Can you work these out from the model? Positions are in its coordinate system, mm. Round coordinates to 2 decimals unless told otherwise and drop trailing zeros. Loops run counter-clockwise (first coordinate to the right, second up) from the corner with the lowest first, then second, coordinate; pieces in that order, holes last. Notation, with made-up numbers: (83.5, -35) - (120.5, -35) arc R27 ccw to (120.5, -9) - close; hole circle Ø4 at (-3.75, 5). An arc over 180 degrees is marked (long way). Answer as CSV lines item,"result".
```python
from build123d import *

# Parameters (mm, degrees)
BOSS_EXTRUDE1_DEPTH   = 10.16
SKETCH2_W             = 76.2
SKETCH2_H             = 10.16
CUT_EXTRUDE1_DEPTH    = 4.572
CHAMFER1_SIZE         = 38.1
CHAMFER1_SIZE2        = 65.991135768
CHAMFER1_PART_2_SIZE  = 38.1
CHAMFER1_PART_2_SIZE2 = 65.991135768
FILLET1_R             = 25.4


with BuildPart() as part:
    # Sketch1 → Boss-Extrude1 (new body)
    with BuildSketch(Plane(origin=(0, 0, 0), x_dir=(0, 0, -1), z_dir=(1, 0, 0))):
        Polygon((-212.802604436, 0), (-212.802604436, 254), (-212.802604436, 279.4), (213.917395564, 279.4), (213.917395564, 254), (213.917395564, 0), (213.917395564, -50.8), (-212.802604436, -50.8), align=None)
        with BuildLine():
            Line((-95.25, 234.95), (95.25, 234.95))
            ThreePointArc((95.25, 234.95), (114.3, 215.9), (95.25, 196.85))
            Line((95.25, 196.85), (-95.25, 196.85))
            ThreePointArc((-95.25, 196.85), (-114.3, 215.9), (-95.25, 234.95))
        make_face(mode=Mode.SUBTRACT)
    extrude(amount=-BOSS_EXTRUDE1_DEPTH)

    # Sketch2 → Cut-Extrude1 (cut)
    with BuildSketch(Plane(origin=(0, 0, 0), x_dir=(0, 0, -1), z_dir=(1, 0, 0))):
        with Locations((-158.192604436, 127)):
            Rectangle(SKETCH2_W, SKETCH2_H)
        with Locations((0.557395564, 127)):
            Rectangle(SKETCH2_W, SKETCH2_H)
        with Locations((159.307395564, 127)):
            Rectangle(SKETCH2_W, SKETCH2_H)
    extrude(amount=-CUT_EXTRUDE1_DEPTH, mode=Mode.SUBTRACT)

    # Chamfer1
    chamfer1_edges = [part.edges().sort_by_distance(p)[0] for p in [
        (-5.08, 279.4, 212.802604436),
        (-5.08, 279.4, -213.917395564),
    ]]
    chamfer1_side = [part.faces().sort_by_distance(p)[0] for p in [
        (-5.08, 279.4, -0.557395564),
    ]]
    chamfer(chamfer1_edges, length=CHAMFER1_SIZE, length2=CHAMFER1_SIZE2, reference=chamfer1_side[0])

    # Chamfer1 part 2
    chamfer1_part_2_edges = [part.edges().sort_by_distance(p)[0] for p in [
        (-5.08, -50.8, -213.917395564),
        (-5.08, -50.8, 212.802604436),
    ]]
    chamfer1_part_2_side = [part.faces().sort_by_distance(p)[0] for p in [
        (-5.08, -50.8, -0.557395564),
    ]]
    chamfer(chamfer1_part_2_edges, length=CHAMFER1_PART_2_SIZE, length2=CHAMFER1_PART_2_SIZE2, reference=chamfer1_part_2_side[0])

    # Fillet1
    fillet1_edges = [part.edges().sort_by_distance(p)[0] for p in [
        (-5.08, -50.8, 174.702604436),
        (-5.08, -50.8, -175.817395564),
        (-5.08, 213.408864232, -213.917395564),
        (-5.08, 15.191135768, -213.917395564),
        (-5.08, 279.4, -175.817395564),
        (-5.08, 279.4, 174.702604436),
        (-5.08, 15.191135768, 212.802604436),
        (-5.08, 213.408864232, 212.802604436),
    ]]
    fillet(fillet1_edges, radius=FILLET1_R)


solid = part.part
```
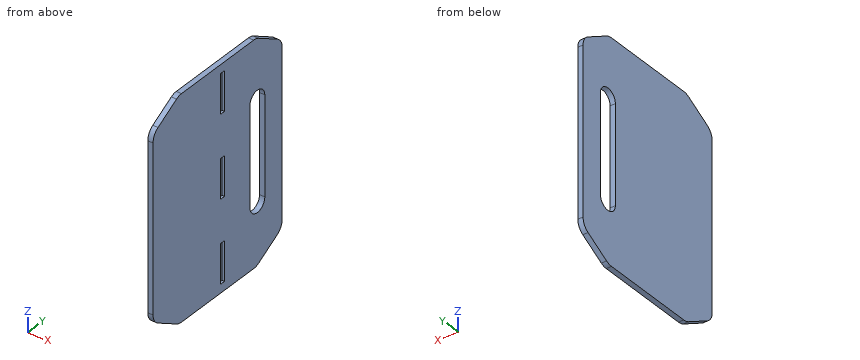
Q1. If I drill on line 1 along Y through (x, z) = (-5.5, 9.5); line 2 along Y through (x, z) = (-1, -142); line 3 along Z through (x, y) = (-6.5, 206), over which ranges is the centre line in solid material (lowest first)? Write a range as [from, to].
Checks:
line 1,"[-50.8, 196.85], [234.95, 279.4]"
line 2,"[-50.8, 121.92], [132.08, 279.4]"
line 3,"[-213.92, -111.53], [111.53, 212.8]"
Q2. Imagine slicing it at B-B (z = 86). Write out the boundary of the cut face in (x, y).
Checks:
outline,"(-10.16, -50.8) - (0, -50.8) - (0, 196.85) - (-10.16, 196.85) - close; (-10.16, 234.95) - (0, 234.95) - (0, 279.4) - (-10.16, 279.4) - close"
Q3. Imagine slicing it at C-C (y = 2.5). Write out the boundary of the cut face in (x, z).
Checks:
outline,"(-10.16, -206.59) - (0, -206.59) - (0, 205.48) - (-10.16, 205.48) - close"
Q4. I'm going to push flat-ended pins straight in: pin 1 Ø11 at (y, z) = (128, 176) entering from +X; pin 2 Ø1 at (x, y) = (-1.5, -6.5) entering from -Z; pin 3 Ø5 at (y, z) = (129, 13.5) entering from +X. Where does each tip first touch, or does it pass through?
Checks:
pin 1,"x = 0"
pin 2,"z = -201.68"
pin 3,"x = -4.57"
Q5. Imagine slicing it at A-A (x = -7). Write out the boundary of the cut face in (y, z), then the cut area to 3 significant figures.
Checks:
outline,"(-50.8, -161.15) arc R25.4 ccw to (-38.1, -183.15) - (9.3, -210.51) arc R25.4 ccw to (22, -213.92) - (206.6, -213.92) arc R25.4 ccw to (219.3, -210.51) - (266.7, -183.15) arc R25.4 ccw to (279.4, -161.15) - (279.4, 160.04) arc R25.4 ccw to (266.7, 182.03) - (219.3, 209.4) arc R25.4 ccw to (206.6, 212.8) - (22, 212.8) arc R25.4 ccw to (9.3, 209.4) - (-38.1, 182.03) arc R25.4 ccw to (-50.8, 160.04) - close; hole (196.85, -95.25) arc R19.05 ccw to (234.95, -95.25) - (234.95, 95.25) arc R19.05 ccw to (196.85, 95.25) - close"
area,"127,000 mm²"
